Design review of the part shown in the three views and the two pictorial views. Dimensions are in mm from the part's minimum x, y and z. A direction names the side the tool comes from. Coordinates: 2 decimals unless noted, no trailing zeros. Loops run counter-clockwise (first coordinate to the right, second up) from the corner with the lowest first, then second, coordinate; pieces in that order, holes last.
Q1. Add section B-B on y = 64. Give the boundary of the cut face in (x, z).
Q2. Draft analysis for pull direction Z (two halves, no side actions). For the marked faces 4, 5 and 6, state which applies: released by +Z, released by -Z, zero draft, split by the parting line, or undercut.
Q3. Add section D-D on y = 48. Give the boundary of the cut face in (x, z).
Q4. Machinability: for the marked faces 1, 2 and 3, which of the approach directions +Z, -Z, +X, -X, +Y, -Y give a long, thin tool a straight path to every point of the face, cutting with its end or side? Answer none if there is none.
Q5. Wall thickness on probe 1 along Z at (x, y) = (152.4, 26.5); probe 2 along Z at (x, y) = (152.4, 45.5); probe 3 along Z at (x, y) = (125, 38): over which ranges is each line inside the solid? List them lowest first.
Q6. Add section A-A on x = 152.4. Give the number of separate pieces and of enclosed holes in the cut face, and give its area (3 significant figures).
Q7. For P1, Ø4, axis at y = 85, z = 52.5, coming from the +X side; P2, Ø5, axis at y = 32, z = 58.5, coming from the +X side; P3, Ø4, axis at y = 83.5, z = 25, coming from the +X side, all flat-tipped, find the tip position at first contact; note any pin that passes through.
Q8. Add section C-C on z = 39.5. Give the boundary of the cut face in (x, y), and give its area (3 significant figures).
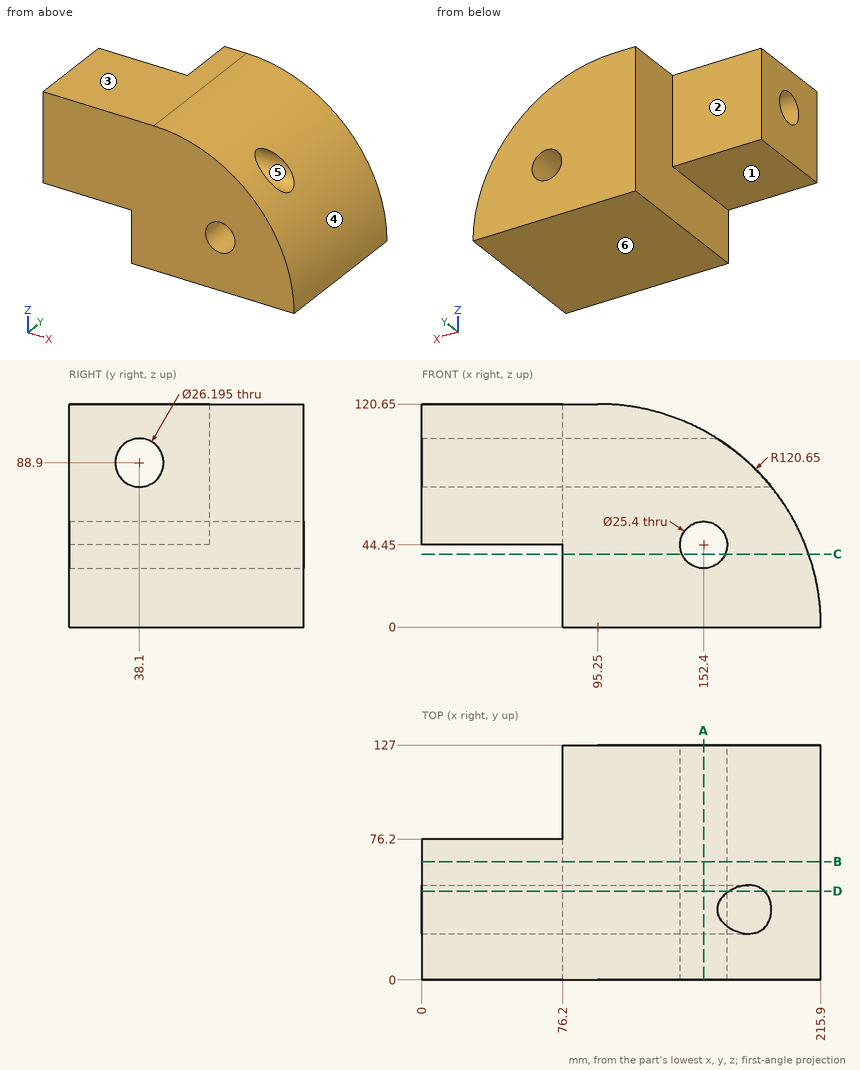
Entries:
1. outline: (0, 44.45) - (76.2, 44.45) - (76.2, 0) - (215.9, 0) arc R120.65 ccw to (95.25, 120.65) - (0, 120.65) - close; hole circle Ø25.4 at (152.4, 44.45)
2. face 4: released by +Z
2. face 5: undercut
2. face 6: released by -Z
3. outline: (0, 44.45) - (76.2, 44.45) - (76.2, 0) - (215.9, 0) arc R120.65 ccw to (185.27, 80.32) - (0, 80.32) - close; (0, 97.48) - (166.35, 97.48) arc R120.65 ccw to (95.25, 120.65) - (0, 120.65) - close; hole circle Ø25.4 at (152.4, 44.45)
4. face 1: -Z, -X, +Y, -Y
4. face 2: +Z, -Z, -X, +Y
4. face 3: +Z, +X, -X, +Y, -Y
5. probe 1: z = 0 to 31.75, 57.15 to 82.82, 94.98 to 106.26
5. probe 2: z = 0 to 31.75, 57.15 to 78.09, 99.71 to 106.26
5. probe 3: z = 0 to 75.8, 102 to 116.92
6. separate pieces: 2
6. enclosed holes: 1
6. area: 9,730 mm2
7. P1: stops at x = 204.82
7. P2: stops at x = 202.12
7. P3: stops at x = 213.69
8. outline: (76.2, 0) - (140.7, 0) - (140.7, 127) - (76.2, 127) - close; (164.1, 0) - (209.25, 0) - (209.25, 127) - (164.1, 127) - close
8. area: 13,900 mm2
